Geometry check sheet. Reference: the model listing, model coordinates, mm. A direction names the side the tool comes from. Give positions to 0.01 mm unless a question says otherwise; leave off trailing zeros. Loops run counter-clockwise (first coordinate to the right, second up) from the corner with the lowest first, then second, coordinate; pieces in that order, holes last. Notation, with made-up numbers: (56, -39.75) - (114, -39.75) arc R7 ccw to (114, -31.75) - close; hole circle Ø3 at (46.5, 25.25). An arc over 180 degrees is marked (long way). Use a Markdown table: item, result. Add a question column.
1. Depth check by flat-ended pin: P1, Ø3, axis at y = 1, z = 0, coming from the -X side. Enter the tip coordinate at first touch or a pass-through.
2. Material ranges on L1, parallel to X at y = 0, z = 2.5; L2, parallel to Y at x = 0, z = -2.7; L3, parallel to Z at x = 21.5, y = 3.5, recorded low to high.
3. Cross-section at A-A on x = 3. Enter the section's corners in (y, z), and give its area (3 significant figures).
4. Cross-section at C-C on z = 2.55. Enter the section's corners in (x, y), and give its area (3 significant figures).
5. Draft check along X on faces 4 (the cylindrical face through (25, 0.1, 2.5)), 5 (the cylindrical face through (-0.54, -2.44, -2.51)), 6 (the cylindrical face through (-5, -0.1, -2.5)). Enter one of: pulls with the +X half, pulls with the -X half, needs draft (parallel to the pull), parting line crosses it, or undercut.
6. Cross-section at D-D on y = 4. Enter the section's corners in (x, z), and give its area (3 significant figures).
7. Cross-section at B-B on y = 0. Enter the section's corners in (x, z), and give its area (3 significant figures).
8. Set-up check for faces 1 (the flat face through (17, 0, -2)), 2 (the flat face through (3, 0, 2)), 3 (the cylindrical face through (17.5, 0.1, 2.5)): record each of +Z, -Z, +X, -X, +Y, -Y from which the full face is reachable in a straight line by a thin tool's end or side.
from build123d import *

# Parameters (mm, degrees)
SKETCH1_R           = 2.5
BOSS_EXTRUDE1_DEPTH = 3
SKETCH2_W           = 20
SKETCH2_H           = 4
CUT_EXTRUDE1_DEPTH  = 28.092434368


with BuildPart() as part:
    # Sketch1 → Boss-Extrude1 (new, symmetric)
    with BuildSketch(Plane.XY):
        with BuildLine():
            Line((0, 5), (20, 5))
            ThreePointArc((20, 5), (25, 0), (20, -5))
            Line((20, -5), (0, -5))
            ThreePointArc((0, -5), (-5, 0), (0, 5))
        make_face()
        Circle(SKETCH1_R, mode=Mode.SUBTRACT)
        with Locations((20, 0)):
            Circle(SKETCH1_R, mode=Mode.SUBTRACT)
    extrude(amount=BOSS_EXTRUDE1_DEPTH, both=True)

    # Sketch2 → Cut-Extrude1 (cut, through all)
    with BuildSketch(Plane(origin=(0, 5, 0), x_dir=(1, 0, 0), z_dir=(0, 1, 0))):
        with Locations((-4, 0)):
            Rectangle(SKETCH2_W, SKETCH2_H)
    cut_extrude1 = extrude(amount=-CUT_EXTRUDE1_DEPTH, mode=Mode.SUBTRACT)

    # Mirror1: Cut-Extrude1 across plane
    add(cut_extrude1.mirror(Plane(origin=(10, 0, 0), x_dir=(0, 0, 1), z_dir=(1, 0, 0))), mode=Mode.SUBTRACT)


solid = part.part
Values found:
| question | item | result |
|---|---|---|
| 1 | P1 | stops at x = 6 |
| 2 | L1 | x = -5 to -2.5, 2.5 to 17.5, 22.5 to 25 |
| 2 | L2 | y = -5 to -2.5, 2.5 to 5 |
| 2 | L3 | z = -3 to -2, 2 to 3 |
| 3 | outline | (-5, -3) - (5, -3) - (5, -2) - (-5, -2) - close; (-5, 2) - (5, 2) - (5, 3) - (-5, 3) - close |
| 3 | area | 20.0 mm2 |
| 4 | outline | (0, -5) - (20, -5) arc R5 ccw to (20, 5) - (0, 5) arc R5 ccw to start; hole circle Ø5 at (0, 0); hole circle Ø5 at (20, 0) |
| 4 | area | 239 mm2 |
| 5 | face 4 | pulls with the +X half |
| 5 | face 5 | undercut |
| 5 | face 6 | pulls with the -X half |
| 6 | outline | (-3, -3) - (23, -3) - (23, -2) - (14, -2) - (14, 2) - (23, 2) - (23, 3) - (-3, 3) - (-3, 2) - (6, 2) - (6, -2) - (-3, -2) - close |
| 6 | area | 84.0 mm2 |
| 7 | outline | (-5, -3) - (-2.5, -3) - (-2.5, -2) - (-5, -2) - close; (-5, 2) - (-2.5, 2) - (-2.5, 3) - (-5, 3) - close; (2.5, -3) - (17.5, -3) - (17.5, -2) - (14, -2) - (14, 2) - (17.5, 2) - (17.5, 3) - (2.5, 3) - (2.5, 2) - (6, 2) - (6, -2) - (2.5, -2) - close; (22.5, -3) - (25, -3) - (25, -2) - (22.5, -2) - close; (22.5, 2) - (25, 2) - (25, 3) - (22.5, 3) - close |
| 7 | area | 72.0 mm2 |
| 8 | face 1 | +X, +Y, -Y |
| 8 | face 2 | -X, +Y, -Y |
| 8 | face 3 | +Z, -Z |
